from build123d import *

# Parameters (mm, degrees)
SKETCH1_R           = 7.9375
SKETCH1_R_2         = 3.2639
SKETCH1_R_3         = 4.191
BOSS_EXTRUDE4_DEPTH = 3.175
FILLET2_R           = 3.81


with BuildPart() as part:
    # Sketch1 → Boss-Extrude4 (new body)
    with BuildSketch(Plane(origin=(0, 0, 0), x_dir=(1, 0, 0), z_dir=(0, 1, 0))):
        with BuildLine():
            ThreePointArc((133.726592386, 29.98785526), (132.627611185, 40.61059676), (122.521356715, 44.06226552))
            Line((122.521356715, 44.06226552), (46.442862481, 25.430137021))
            ThreePointArc((46.442862481, 25.430137021), (36.958837973, 28.991331503), (30.193743977, 21.450619984))
            Line((30.193743977, 21.450619984), (-3.247611444, 13.260609947))
            ThreePointArc((-3.247611444, 13.260609947), (-13.515826194, -1.926966151), (0.587616374, -13.639848359))
            Line((0.587616374, -13.639848359), (108.971460257, -8.970579339))
            ThreePointArc((108.971460257, -8.970579339), (113.459157615, -7.540771363), (116.60566957, -4.036025875))
            Line((116.60566957, -4.036025875), (133.726592386, 29.98785526))
        make_face()
        with Locations(Location((0, 0, 0), (0, 0, 270))):
            Circle(SKETCH1_R, mode=Mode.SUBTRACT)
        with BuildLine():
            Line((41.984168993, -4.864970405), (12.189591197, -6.148546389))
            ThreePointArc((12.189591197, -6.148546389), (13.515826194, 1.926966151), (9.985636063, 9.310092839))
            Line((9.985636063, 9.310092839), (32.042893317, 14.712061629))
            ThreePointArc((32.042893317, 14.712061629), (34.888474765, 12.337435423), (38.450716367, 11.314391845))
            Line((38.450716367, 11.314391845), (41.984168993, -4.864970405))
        make_face(mode=Mode.SUBTRACT)
        with BuildLine():
            Line((69.18664036, 23.808811963), (47.410466333, -5.902378846))
            Line((47.410466333, -5.902378846), (43.413738486, 12.398279038))
            ThreePointArc((43.413738486, 12.398279038), (46.36017499, 14.994407118), (47.916850432, 18.599699151))
            Line((47.916850432, 18.599699151), (69.18664036, 23.808811963))
        make_face(mode=Mode.SUBTRACT)
        with Locations(Location((108.585, 0, 0), (0, 0, 270))):
            Circle(SKETCH1_R_2, mode=Mode.SUBTRACT)
        with Locations(Location((39.094708942, 20.270167566, 0), (0, 0, 270))):
            Circle(SKETCH1_R_2, mode=Mode.SUBTRACT)
        with BuildLine():
            Line((99.924218758, -2.368863331), (54.876229285, -4.309569382))
            Line((54.876229285, -4.309569382), (78.030840873, 27.282347644))
            Line((78.030840873, 27.282347644), (100.723144875, 4.337266328))
            ThreePointArc((100.723144875, 4.337266328), (99.66914772, 1.062178575), (99.924218758, -2.368863331))
        make_face(mode=Mode.SUBTRACT)
        with BuildLine():
            Line((84.823475635, 27.638376771), (114.98908268, 35.026134276))
            ThreePointArc((114.98908268, 35.026134276), (117.570132445, 27.752761279), (124.58688197, 24.538885311))
            Line((124.58688197, 24.538885311), (115.260501822, 6.004858086))
            ThreePointArc((115.260501822, 6.004858086), (110.126982004, 8.845503757), (104.335087932, 7.90941797))
            Line((104.335087932, 7.90941797), (84.823475635, 27.638376771))
        make_face(mode=Mode.SUBTRACT)
        with Locations(Location((124.877763158, 34.440613651, 0), (0, 0, 270))):
            Circle(SKETCH1_R_3, mode=Mode.SUBTRACT)
    extrude(amount=-BOSS_EXTRUDE4_DEPTH)

    # Fillet1
    # a fillet whose section is not a circle: 7.62 mm, written as the material it adds along each edge
    with BuildSketch(Plane(origin=(115.260501822, 0, -6.004858086), x_dir=(-0.8680919950979666, 0, -0.4964033521712276), z_dir=(0, -1, 0))) as fillet1_piece_1:
        with BuildLine():
            Bezier((5.628236023, 0), (0.097286133, 1.825453133), (0.407253439, 7.641603586), weights=[1, 1, 1])
            Line((0.407253439, 7.641603586), (0, 0))
            ThreePointArc((0, 0), (2.814118011, 0.452389282), (5.628236023, 0))
        make_face()
    extrude(amount=3.175)
    with BuildSketch(Plane(origin=(124.58688197, 0, -24.538885311), x_dir=(-0.9406523774093201, 0, -0.3393716323946274), z_dir=(0, -1, 0))) as fillet1_piece_2:
        with BuildLine():
            Bezier((6.173495259, 0), (0.234745196, -1.947499202), (0.982676409, -8.152505596), weights=[1, 1, 1])
            Line((0.982676409, -8.152505596), (0, 0))
            ThreePointArc((0, 0), (3.08674763, -0.493198872), (6.173495259, 0))
        make_face()
    extrude(amount=3.175)
    with BuildSketch(Plane(origin=(114.98908268, 0, -35.026134276), x_dir=(-0.9712953632492297, 0, 0.23787668513443497), z_dir=(0, -1, 0))) as fillet1_piece_3:
        with BuildLine():
            Bezier((7.418766675, 0), (1.629858857, 0), (0.077760385, -5.576956522), weights=[1, 1, 1])
            ThreePointArc((0.077760385, -5.576956522), (0.439489428, -2.782892503), (0, 0))
            Line((0, 0), (7.418766675, 0))
        make_face()
    extrude(amount=3.175)
    with BuildSketch(Plane(origin=(9.985636063, 0, -9.310092839), x_dir=(0.4554657293432797, 0, 0.8902533175415829), z_dir=(0, -1, 0))) as fillet1_piece_4:
        with BuildLine():
            Bezier((7.480452048, 0), (0.473095274, -1.996096811), (2.153427849, -9.085803001), weights=[1, 1, 1])
            Line((2.153427849, -9.085803001), (0, 0))
            ThreePointArc((0, 0), (3.740226024, -0.522326142), (7.480452048, 0))
        make_face()
    extrude(amount=3.175)
    with BuildSketch(Plane(origin=(99.924218758, 0, 2.368863331), x_dir=(0.01787605144618897, 0, -0.9998402106260246), z_dir=(0, -1, 0))) as fillet1_piece_5:
        with BuildLine():
            Bezier((5.046610766, 0), (-0.091794663, -1.504663887), (-0.417829547, -6.848906118), weights=[1, 1, 1])
            Line((-0.417829547, -6.848906118), (0, 0))
            ThreePointArc((0, 0), (2.523305383, -0.361848581), (5.046610766, 0))
        make_face()
    extrude(amount=3.175)
    with BuildSketch(Plane(origin=(12.189591197, 0, 6.148546389), x_dir=(0.9990733095506228, 0, -0.043040935672514394), z_dir=(0, -1, 0))) as fillet1_piece_6:
        with BuildLine():
            Bezier((9.337508644, 0), (2.051395042, 0), (1.725151149, -7.27880597), weights=[1, 1, 1])
            ThreePointArc((1.725151149, -7.27880597), (1.370821683, -3.518943481), (0, 0))
            Line((0, 0), (9.337508644, 0))
        make_face()
    extrude(amount=3.175)

    # Fillet2
    fillet2_edges = [part.edges().sort_by_distance(p)[0] for p in [
        (104.335087932, -1.5875, -7.90941797),
        (100.723144875, -1.5875, -4.337266328),
        (84.823475635, -1.5875, -27.638376771),
        (69.18664036, -1.5875, -23.808811963),
        (41.984168993, -1.5875, 4.864970405),
        (32.042893317, -1.5875, -14.712061629),
        (47.916850432, -1.5875, -18.599699151),
        (38.450716367, -1.5875, -11.314391845),
        (43.413738486, -1.5875, -12.398279038),
        (54.876229285, -1.5875, 4.309569382),
        (47.410466333, -1.5875, 5.902378846),
        (78.030840873, -1.5875, -27.282347644),
        (30.193743977, -1.5875, -21.450619984),
        (46.442862481, -1.5875, -25.430137021),
    ]]
    fillet(fillet2_edges, radius=FILLET2_R)


solid = part.part
Part model, mm, in its own coordinate system. A direction names the side the tool comes from. Coordinates: 2 decimals unless noted, no trailing zeros. Use a Markdown table: item, result. Add a question column.
Item 1: Pull direction Z, two halves, no side cores. Call faces 3 (the cylindrical face through (31.69, -1.61, -14.21)), 4 (the cylindrical face through (37, -2, -29)), 5 (the flat face through (62, -3.175, -9)): +Z half, -Z half, draft (parallel to the pull), parting line (faces both ways), or undercut.
Item 2: Which spindle directions (+Z, -Z, +X, -X, +Y, -Y) get a long thin tool onto all of the face, cutting with end or side? Do faces 1 (the cylindrical face through (48.421, -1.61, -18.285)), 2 (the flat face through (62, 0, -9)). Say none if no direction does.
Item 3: Band-saw the part on A-A on y = -2. Give the number of separate pieces and of enclosed holes in the cut face, plus the area to 3 significant figures.
Item 4: Probe probe 1 along X at (y, z) = (-1.55, 0); probe 2 along X at (y, z) = (-2.1, -7); probe 3 along Z at (x, y) = (89, -1.1). List the from-to ranges inside material, lowest first.
Geometry says:
| question | item | result |
|---|---|---|
| 1 | face 3 | undercut |
| 1 | face 4 | -Z half |
| 1 | face 5 | draft |
| 2 | face 1 | +Y, -Y |
| 2 | face 2 | +Z, -Z, +X, -X, +Y |
| 3 | separate pieces | 1 |
| 3 | enclosed holes | 8 |
| 3 | area | 3,110 mm² |
| 4 | probe 1 | -13.65 to -7.94, 7.94 to 13.76, 40.92 to 47.21, 51.46 to 58.83, 98.68 to 105.32, 111.85 to 118.64 |
| 4 | probe 2 | -11.72 to -3.74, 3.74 to 13.45, 39.39 to 44.59, 56.87 to 63.17, 98.09 to 122.16 |
| 4 | probe 3 | -35.85 to -27.51, -23.57 to -16.19, 2.84 to 9.83 |
